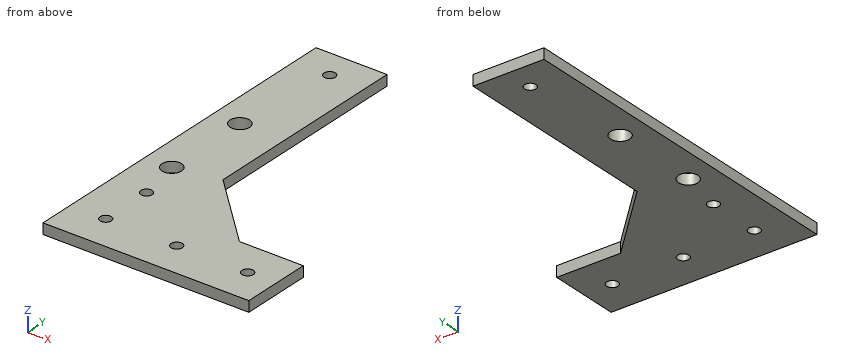
```python
from build123d import *

# Parameters (mm, degrees)
EXTRUDE1_DEPTH     = 3
SKETCH2_R          = 1.6
SKETCH2_R_2        = 2.75
CUT_EXTRUDE1_DEPTH = 3


with BuildPart() as part:
    # Sketch1 → Extrude1 (new body)
    with BuildSketch(Plane.XY):
        Polygon((-195.489923187, -7.502951786), (-195.489923187, -27.502951786), (-253.489921235, -27.502951786), (-253.489921235, 72.709593142), (-233.489921235, 72.709593142), (-233.489921235, 12.497048214), (-213.489921235, -7.502951786), align=None)
    extrude(amount=EXTRUDE1_DEPTH)

    # Sketch2 → Cut-Extrude1 (cut)
    with BuildSketch(Plane.XY.offset(3)):
        with Locations((-203.489923187, -17.502951786)):
            Circle(SKETCH2_R)
        with Locations((-223.489923187, -17.502951786)):
            Circle(SKETCH2_R)
        with Locations((-243.489923187, -17.502951786)):
            Circle(SKETCH2_R)
        with Locations((-243.489923187, -2.502951786)):
            Circle(SKETCH2_R)
        with Locations((-245.989921235, 9.997448214)):
            Circle(SKETCH2_R_2)
        with Locations((-245.989921235, 34.997448214)):
            Circle(SKETCH2_R_2)
        with Locations((-243.489923187, 64.709593142)):
            Circle(SKETCH2_R)
    extrude(amount=-CUT_EXTRUDE1_DEPTH, mode=Mode.SUBTRACT)


solid = part.part
```
Geometry check sheet. Reference: the model listing, model coordinates, mm. Give positions to 0.01 mm unless a question says otherwise; leave off trailing zeros. Write each loop counter-clockwise with the first axis right and the second up, starting at its lowest first coordinate (ties: lowest second). Pieces come first, ordered by that corner, then holes. Notation, with made-up numbers: (72, 23.25) -> (95, 23.25) arc R21 cw to (95, 35.25) -> close; hole circle Ø3 at (-5, 36). An arc over 180 degrees is marked (long way). Use one line per item in the form item = value.
Item 1: Depth check by flat-ended pin: pin 1 Ø1.5 at (x, z) = (-207, 2) entering from +Y; pin 2 Ø1.9 at (x, y) = (-223.49, -17.5) entering from -Z; pin 3 Ø6.5 at (x, y) = (-245.99, 35) entering from -Z. Enter the tip coordinate at first touch or a pass-through.
Results list:
pin_1 = -7.5
pin_2 = through
pin_3 = 0
Item 2: Sectioned sample at D-D on x = -207.5. Enter the section's corners in (y, z).
Results list:
outline = (-27.5, 0) -> (-7.5, 0) -> (-7.5, 3) -> (-27.5, 3) -> close
Item 3: Sectioned sample at A-A on x = -247. Enter the section's corners in (y, z).
Results list:
outline = (-27.5, 0) -> (7.44, 0) -> (7.44, 3) -> (-27.5, 3) -> close; (12.56, 0) -> (32.44, 0) -> (32.44, 3) -> (12.56, 3) -> close; (37.56, 0) -> (72.71, 0) -> (72.71, 3) -> (37.56, 3) -> close
Item 4: Sectioned sample at C-C on y = 48. Enter the section's corners in (x, z).
Results list:
outline = (-253.49, 0) -> (-233.49, 0) -> (-233.49, 3) -> (-253.49, 3) -> close
Item 5: Scan lines: line 1 (X direction, y = 64.5, z = 2.8); line 2 (Y direction, x = -248, z = 1.7); line 3 (Y direction, x = -203.5, z = 0.2). Record each from-to range of solid material in increasing order.
Results list:
line_1 = -253.49 to -245.08, -241.9 to -233.49
line_2 = -27.5 to 8.12, 11.87 to 33.12, 36.87 to 72.71
line_3 = -27.5 to -19.1, -15.9 to -7.5
Item 6: Sectioned sample at B-B on z = 1.4. Enter the section's corners in (x, y), plus the area to 3 significant figures.
Results list:
outline = (-253.49, -27.5) -> (-195.49, -27.5) -> (-195.49, -7.5) -> (-213.49, -7.5) -> (-233.49, 12.5) -> (-233.49, 72.71) -> (-253.49, 72.71) -> close; hole circle Ø5.5 at (-245.99, 10); hole circle Ø5.5 at (-245.99, 35); hole circle Ø3.2 at (-243.49, -17.5); hole circle Ø3.2 at (-243.49, -2.5); hole circle Ø3.2 at (-243.49, 64.71); hole circle Ø3.2 at (-223.49, -17.5); hole circle Ø3.2 at (-203.49, -17.5)
area = 2,880 mm2
